Input: part model. Units: mm. Frame: model coordinates. Face numbers are marked on the shaded views. A direction names the side the tool comes from. Coordinates: 2 decimals unless noted, no trailing zeros. Loops run counter-clockwise (first coordinate to the right, second up) from the corner with the lowest first, then second, coordinate; pieces in that order, holes last. Notation, with made-up numbers: M 25,-38.5 L 70,-38.5 A20 ccw 70,-18.5 Z; hole C 16.25,72 d1. An arc over 180 degrees is marked long. Use a Markdown table: item, result. Add a question column.
1. Section A-A on x = 4.5. Output: boundary loops of the cut face in (y, z), then the cut area to 3 significant figures.
2. Set-up query: the marked faces 4, 5 and 6. Return all of +Z, -Z, +X, -X, +Y, -Y with unobstructed straight access to the full face (end or side cutting, diameter ignored); none if empty.
3. Section C-C on x = 2.5. Output: boundary loops of the cut face in (y, z), then the cut area to 3 significant figures.
4. Draft query along Y for the marked faces 1, 2 and 3. Return one class per face: +Y half, -Y half, draft (parallel to the pull), parting line (faces both ways), or undercut.
5. Line query: L1, parallel to Y at x = 6.5, z = -16; L2, parallel to Z at x = 7.25, y = -27.5; L3, parallel to X at y = -30.25, z = -12.75. Output: solid intervals per line, ascending. Write a range as [from, to].
6. Section D-D on y = -30.25. Output: boundary loops of the cut face in (x, z).
7. Pin query (flat end, axial travel): pin 1 (2 mm diameter, centred on y = -30.5, z = -18, fed in from -X); pin 2 (3 mm diameter, centred on x = 3.74, y = -31.83, fed in from +Z); pin 3 (2.5 mm diameter, centred on x = 4.5, z = -15, fed in from +Y). Return the tip coordinate at first contact, or that it passes through.
8. Section B-B on z = -11.5. Output: boundary loops of the cut face in (x, y), then the cut area to 3 significant figures.
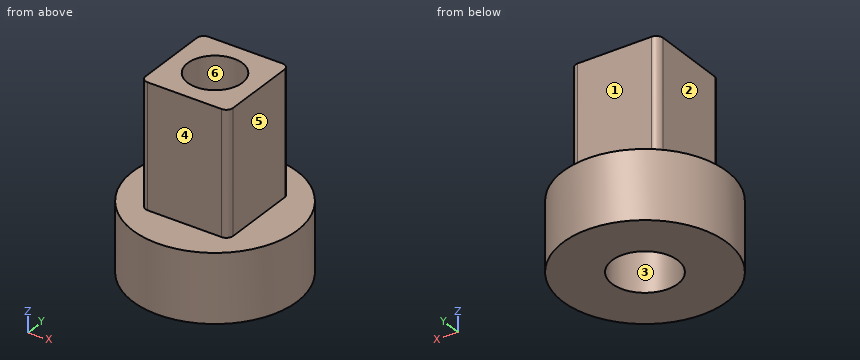
```python
from build123d import *

# Parameters (mm, degrees)
SKETCH1_R           = 6
SKETCH1_R_2         = 2.4
BOSS_EXTRUDE1_DEPTH = 5
BOSS_EXTRUDE2_DEPTH = 9
CUT_EXTRUDE1_REACH  = 16
SKETCH3_R           = 1
SKETCH4_R           = 2
CUT_EXTRUDE2_DEPTH  = 7


with BuildPart() as part:
    # Sketch1 → Boss-Extrude1 (new body)
    with BuildSketch(Plane.XY.offset(-23.465471353)):
        with Locations((3.740457308, -31.828386779)):
            Circle(SKETCH1_R)
        with Locations((3.740457308, -31.828386779)):
            Circle(SKETCH1_R_2, mode=Mode.SUBTRACT)
    extrude(amount=BOSS_EXTRUDE1_DEPTH)

    # Sketch2 → Boss-Extrude2 (add)
    with BuildSketch(Plane.XY.offset(-18.465471353)):
        with BuildLine():
            Line((6.440457308, -28.628386779), (1.040457308, -28.628386779))
            ThreePointArc((1.040457308, -28.628386779), (0.686903918, -28.774833388), (0.540457308, -29.128386779))
            Line((0.540457308, -29.128386779), (0.540457308, -34.528386779))
            ThreePointArc((0.540457308, -34.528386779), (0.686903918, -34.881940169), (1.040457308, -35.028386779))
            Line((1.040457308, -35.028386779), (6.440457308, -35.028386779))
            ThreePointArc((6.440457308, -35.028386779), (6.794010699, -34.881940169), (6.940457308, -34.528386779))
            Line((6.940457308, -34.528386779), (6.940457308, -29.128386779))
            ThreePointArc((6.940457308, -29.128386779), (6.794010699, -28.774833388), (6.440457308, -28.628386779))
        make_face()
    extrude(amount=BOSS_EXTRUDE2_DEPTH)

    # Sketch3 → Cut-Extrude1 (cut, up to next)
    with BuildSketch(Plane.XY.offset(-9.465471353), mode=Mode.PRIVATE) as cut_extrude1_sk1:
        with Locations((3.740457264, -31.828386779)):
            Circle(SKETCH3_R)
    cut_extrude1_tool1 = extrude(cut_extrude1_sk1.sketch, amount=-CUT_EXTRUDE1_REACH, mode=Mode.PRIVATE) & part.part
    add(cut_extrude1_tool1.solids().sort_by_distance((3.740457, -31.828387, -9.465471))[0], mode=Mode.SUBTRACT)

    # Sketch4 → Cut-Extrude2 (cut)
    with BuildSketch(Plane.XY.offset(-9.465471353)):
        with Locations((3.740457264, -31.828386779)):
            Circle(SKETCH4_R)
    extrude(amount=-CUT_EXTRUDE2_DEPTH, mode=Mode.SUBTRACT)


solid = part.part
```
Answers below:
| question | item | result |
|---|---|---|
| 1 | outline | M -37.78,-23.47 L -34.11,-23.47 L -34.11,-18.47 L -32.48,-18.47 L -32.48,-16.47 L -33.68,-16.47 L -33.68,-9.47 L -35.03,-9.47 L -35.03,-18.47 L -37.78,-18.47 Z; M -31.18,-18.47 L -29.55,-18.47 L -29.55,-23.47 L -25.88,-23.47 L -25.88,-18.47 L -28.63,-18.47 L -28.63,-9.47 L -29.98,-9.47 L -29.98,-16.47 L -31.18,-16.47 Z |
| 1 | area | 65.8 mm² |
| 2 | face 4 | +Z, +X, -X, -Y |
| 2 | face 5 | +Z, +X, +Y, -Y |
| 2 | face 6 | +Z |
| 3 | outline | M -37.7,-23.47 L -33.88,-23.47 L -33.88,-18.47 L -29.77,-18.47 L -29.77,-23.47 L -25.96,-23.47 L -25.96,-18.47 L -28.63,-18.47 L -28.63,-9.47 L -30.26,-9.47 L -30.26,-16.47 L -33.4,-16.47 L -33.4,-9.47 L -35.03,-9.47 L -35.03,-18.47 L -37.7,-18.47 Z |
| 3 | area | 73.8 mm² |
| 4 | face 1 | +Y half |
| 4 | face 2 | draft |
| 4 | face 3 | undercut |
| 5 | L1 | y = [-35.02, -28.63] |
| 5 | L2 | z = [-23.47, -18.47] |
| 5 | L3 | x = [0.54, 2.51], [4.97, 6.94] |
| 6 | outline | M -2.05,-23.47 L 1.93,-23.47 L 1.93,-18.47 L 5.55,-18.47 L 5.55,-23.47 L 9.53,-23.47 L 9.53,-18.47 L 6.94,-18.47 L 6.94,-9.47 L 4.97,-9.47 L 4.97,-16.47 L 2.51,-16.47 L 2.51,-9.47 L 0.54,-9.47 L 0.54,-18.47 L -2.05,-18.47 Z |
| 7 | pin 1 | stops at x = -2.24 |
| 7 | pin 2 | stops at z = -16.47 |
| 7 | pin 3 | stops at y = -28.63 |
| 8 | outline | M 0.54,-34.53 A0.5 ccw 1.04,-35.03 L 6.44,-35.03 A0.5 ccw 6.94,-34.53 L 6.94,-29.13 A0.5 ccw 6.44,-28.63 L 1.04,-28.63 A0.5 ccw 0.54,-29.13 Z; hole C 3.74,-31.83 d4 |
| 8 | area | 28.2 mm² |
